Here's how the part is built. I have some questions about the finished solid (model axes, mm). Face numbers are marked on the shaded views. A direction names the side the tool comes from. Give positions to 0.01 mm unless a question says otherwise; leave off trailing zeros. Write each loop counter-clockwise with the first axis right and the second up, starting at its lowest first coordinate (ties: lowest second). Pieces come first, ordered by that corner, then holes. Notation, with made-up numbers: (-2, -23.75) -> (34, -23.75) arc R16 ccw to (34, -10.75) -> close; hole circle Ø8 at (-15, -22.5). An arc over 180 degrees is marked (long way). Return JSON: item names as keys, results as strings.
Autodesk Inventor part; units mm, degrees
ref_plane "YZ Plane" through (0, 0, 0) normal (1, 0, 0) x (0, 1, 0)
ref_plane "XZ Plane" through (0, 0, 0) normal (0, 1, 0) x (-1, 0, 0)
ref_plane "XY Plane" through (0, 0, 0) normal (0, 0, 1) x (1, 0, 0)
sketch "Sketch1" plane through (0, 0, 0) normal (0, 1, 0) x (-1, 0, 0)
  circle A0 centre (0, 0) radius 16
  dimension "d74" = 32
extrude "Extrusion3" add sketch "Sketch1" along normal blind 3
sketch "Sketch4" plane through (0, 3, 0) normal (0, 1, 0) x (1, 0, 0)
  circle A0 centre (0, 0) radius 12.5
  line L0 (-4.3909, 10.9342) -> (-4.3909, 17.3914)
  line L1 (-4.3909, 17.3914) -> (-7.1862, 17.3914)
  line L2 (-7.1862, 17.3914) -> (-7.1862, 9.3059)
  line L3 (-7.1862, 9.3059) -> (-4.3909, 9.3059)
  line L4 (-4.3909, 9.3059) -> (-4.3909, 10.9342)
  dimension "d77" = 25
extrude "Extrusion4" cut sketch "Sketch4" against normal through all
chamfer "Chamfer3" distance 3 angle 45 1 edges at (-4.3909, 3, -13.5446)
chamfer "Chamfer4" distance 3 angle 45 1 edges at (-7.1862, 0, -12.2616)
properties part number "reverse gear piston gear"
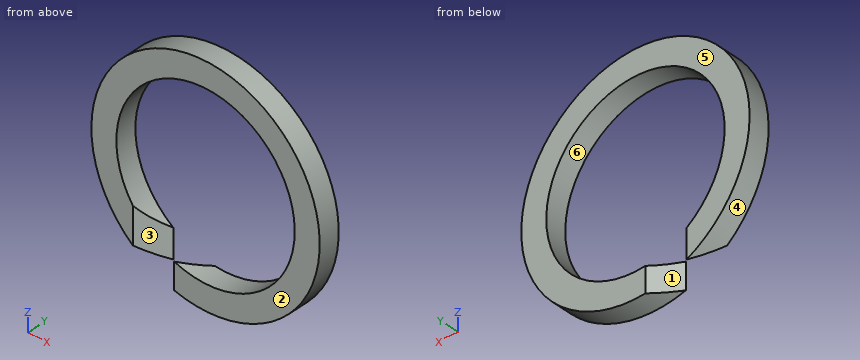
1. If I drill on line 1 (X direction, y = 1.7, z = 0); line 2 (X direction, y = 1.8, z = -3), over which ranges is the centre line in solid material (lowest first)? Write a range as [from, to].
Taken from the geometry:
{"line 1": "x = [-16, -12.5], [12.5, 16]", "line 2": "x = [-15.72, -12.13], [12.13, 15.72]"}
2. Suppose I cut it at B-B, the plane x = 0. List the corners of the cut face in (y, z) for me.
Taken from the geometry:
{"outline": "(0, -16) -> (3, -16) -> (3, -12.5) -> (0, -12.5) -> close; (0, 12.5) -> (3, 12.5) -> (3, 16) -> (0, 16) -> close"}
3. If we mould it in two halves opening along Z, with no side actions, what happens to the marked faces 4, 5 and 6? For each: released by +Z, released by -Z, zero draft, split by the parting line, or undercut.
Taken from the geometry:
{"face 4": "split by the parting line", "face 5": "zero draft", "face 6": "undercut"}
4. Suppose I cut it at A-A, the plane z = 0. List the corners of the cut face in (x, y) for me.
Taken from the geometry:
{"outline": "(-16, 0) -> (-12.5, 0) -> (-12.5, 3) -> (-16, 3) -> close; (12.5, 0) -> (16, 0) -> (16, 3) -> (12.5, 3) -> close"}
5. Which directions (+Z, -Z, +X, -X, +Y, -Y) give clear straight access to the entire face, cutting with the end or side of a thin tool? Please do the marked faces 1, 2 and 3.
Taken from the geometry:
{"face 1": "-Z, +Y", "face 2": "+Z, -Z, +X, -X, -Y", "face 3": "-Z, -Y"}
6. Suppose I cut it at D-D, the plane y = 2. List the corners of the cut face in (x, z) for me.
Taken from the geometry:
{"outline": "(-8.19, -13.75) -> (-8.19, -9.45) arc R12.5 cw (long way) to (-2.39, -12.27) -> (-2.39, -15.82) arc R16 ccw (long way) to start"}
